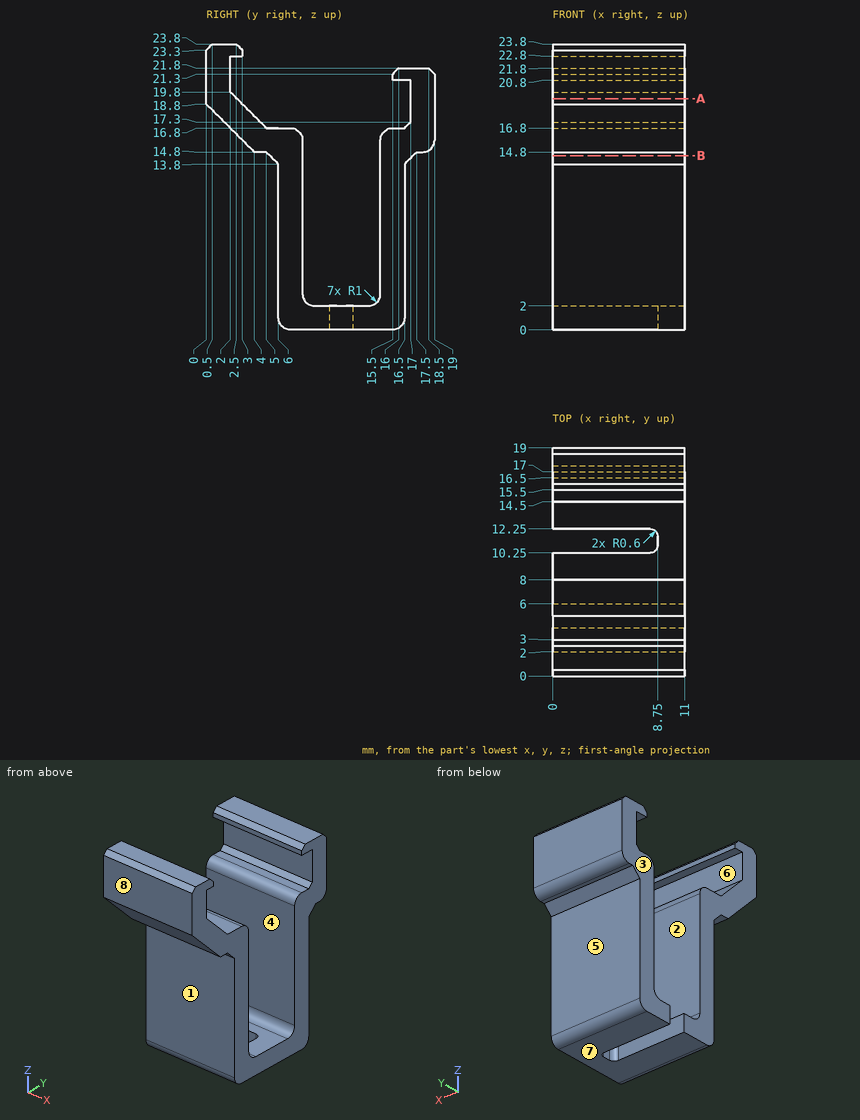
Input: dimensioned drawing with shaded views. Units: mm. Origin: part minimum x, y, z. A direction names the side the tool comes from. Coordinates: 2 decimals unless noted, no trailing zeros. Order: outer loops, then holes, each group sorted by start corner. A loop starts at its lowest first (then second) coordinate and runs counter-clockwise, first axis right, second up. Notation, with made-up numbers: (-28.5, 51) - (6.5, 51) arc R20 cw to (6.5, 78) - close; hole circle Ø5 at (-36, 62.25). An arc over 180 degrees is marked (long way). Return JSON: item names as keys, results as strings. Group by question number.
1. Pull-direction query (Y, two-part tool) for the marked faces 1, 2 and 3; classes: pulls with the +Y half, pulls with the -Y half, needs draft (parallel to the pull), parting line crosses it, or undercut.
2. Pin query (flat end, axial travel): pin 1 (0.5 mm diameter, centred on x = 5.5, y = 4.5, fed in from -Z); pin 2 (6 mm diameter, centred on x = 9.5, y = 15.5, fed in from +Z); pin 3 (1.6 mm diameter, centred on x = 5.5, y = 6, fed in from +Z); pin 4 (5 mm diameter, centred on y = 11, z = 8.5, fed in from +X). Return the tip coordinate at first contact, or that it passes through.
3. Cut plane B-B (z = 14.5). Output: boundary loops of the cut face in (x, y), plus the area to 3 significant figures.
4. Set-up query: the marked faces 4, 5, 6, 7 and 8. Return all of +Z, -Z, +X, -X, +Y, -Y with unobstructed straight access to the full face (end or side cutting, diameter ignored); none if empty.
5. Cut plane A-A (z = 19.25). Output: boundary loops of the cut face in (x, y), plus the area to 4 significant figures.
6. Material intervals for line 1 along Y through (x, z) = (4.5, 7.5); line 2 along Z through (x, y) = (3, 12.75); line 3 along Z through (x, y) = (1.75, 4.5), sorted ascending. Write a range as [from, to].
Resolved:
{
 "1": {"face 1": "pulls with the -Y half", "face 2": "undercut", "face 3": "needs draft"},
 "2": {"pin 1": "stops at z = 14.8", "pin 2": "stops at z = 21.8", "pin 3": "stops at z = 16.8", "pin 4": "passes through"},
 "3": {"outline": "(0, 5.3) - (11, 5.3) - (11, 8) - (0, 8) - close; (0, 14.5) - (11, 14.5) - (11, 17.2) - (0, 17.2) - close", "area": "59.4 mm²"},
 "4": {"face 4": "+Z, +X, -X", "face 5": "-Z, +X, -X, +Y", "face 6": "+X, -X", "face 7": "-Z, +X, -X, +Y, -Y", "face 8": "+Z, -Z, +X, -X, -Y"},
 "5": {"outline": "(0, 0) - (11, 0) - (11, 2.55) - (0, 2.55) - close; (0, 17) - (11, 17) - (11, 19) - (0, 19) - close", "area": "50.05 mm²"},
 "6": {"line 1": "y = [6, 8], [14.5, 16.5]", "line 2": "z = [0, 2]", "line 3": "z = [14.8, 17.3]"}
}
